The model under review builds one solid part; all positions refer to its coordinate system, in mm. A direction names the side the tool comes from. Coordinates: 2 decimals unless noted, no trailing zeros. Order: outer loops, then holes, each group sorted by start corner. A loop starts at its lowest first (then second) coordinate and runs counter-clockwise, first axis right, second up. Notation, with made-up numbers: M -1,15 L 29,15 A32 cw 29,44 Z; hole C 75.5,9 d9. An arc over 180 degrees is marked long. Answer in a Markdown table with one row per item.
from build123d import *

# Parameters (mm, degrees)
F1_DEPTH  = 9.398
F2_W      = 76.2
F2_H      = 33.274
F3_DEPTH  = 9.398
F4_W      = 76.2
F4_H      = 29.7886691538
F5_DEPTH  = 63.754
F6_SIZE   = 11.43
F7_W      = 76.2
F7_H      = 20.574
F8_DEPTH  = 10.414
F9_R      = 14.224
F10_DEPTH = 58.928


with BuildPart() as f1:
    # F0 (on Top) → F1 (new body)
    with BuildSketch(Plane.XY):
        Polygon((-69.8201261675, 38.4550108689), (-69.8201261675, 21.1263484053), (6.3798738325, 21.1263484053), (6.3798738325, 38.4550108689), (-27.0211261675, 84.4290108689), (-36.4191261675, 84.4290108689), align=None)
    extrude(amount=F1_DEPTH)

    # F2 (on face) → F3 (join)
    with BuildSketch(Plane.XZ.offset(-21.1263484053)):
        with Locations((-31.7201261675, -16.637)):
            Rectangle(F2_W, F2_H)
    extrude(amount=-F3_DEPTH)

    # F4 (on face) → F5 (join)
    with BuildSketch(Plane.XZ.offset(-21.1263484053)):
        with Locations((-31.7201261675, -18.3796654231)):
            Rectangle(F4_W, F4_H)
    extrude(amount=F5_DEPTH)

    # F6
    f6_edges = [f1.edges().sort_by_distance(p)[0] for p in [
        (6.379874, -10.750652, -3.485331),
        (-69.820126, -10.750652, -3.485331),
    ]]
    chamfer(f6_edges, length=F6_SIZE)

    # F7 (on face) → F8 (join)
    with BuildSketch(Plane(origin=(0, 0, -33.274), x_dir=(1, 0, 0), z_dir=(0, 0, -1))):
        with Locations((-31.7201261675, 0.5906515947)):
            Rectangle(F7_W, F7_H)
    extrude(amount=F8_DEPTH)

    # F9 (on face) → F10 (cut)
    with BuildSketch(Plane.XY.offset(-3.4853308462)):
        with Locations((-31.7201261675, -10.7506515947)):
            Circle(F9_R)
    extrude(amount=-F10_DEPTH, mode=Mode.SUBTRACT)


solid = f1.part
(1) Take a section at A-A (y = -20.5). Write out the cut boundary in (x, z), then the cut area to 3 significant figures.
Report:
| item | result |
|---|---|
| outline | M -69.82,-33.27 L -42.08,-33.27 L -42.08,-3.49 L -58.39,-3.49 L -69.82,-14.92 Z; M -21.36,-33.27 L 6.38,-33.27 L 6.38,-14.92 L -5.05,-3.49 L -21.36,-3.49 Z |
| area | 1,520 mm^2 |
(2) Machinability: for faces 5 (the flat face through (-32, 9.696, -38)), 6 (the flat face through (-44, -3, -3.485)), 7 (the flat face through (-6, -10.878, -38)), which of the approach directions +Z, -Z, +X, -X, +Y, -Y give a long, thin tool a straight path to every point of the face, cutting with its end or side? Answer none if there is none.
Report:
| item | result |
|---|---|
| face 5 | -Z, +X, -X, +Y |
| face 6 | +Z, +X, -X, -Y |
| face 7 | -Z, +X, -X, -Y |
(3) Take a section at B-B (z = 6.5). Write out the cut boundary in (x, y).
Report:
| item | result |
|---|---|
| outline | M -69.82,21.13 L 6.38,21.13 L 6.38,38.46 L -27.02,84.43 L -36.42,84.43 L -69.82,38.46 Z |
(4) To check wall thickness, follow line 1 (X direction, y = -10.5, z = -27.5); line 2 (Z direction, x = -54, y = -30.5); line 3 (Y direction, x = -15.5, z = -32). State the ranges of each line that lie inside material, in increasing order. Write a range as [from, to].
Report:
| item | result |
|---|---|
| line 1 | [-69.82, -45.94], [-17.5, 6.38] |
| line 2 | [-33.27, -3.49] |
| line 3 | [-42.63, 30.52] |
(5) The part is to be moulded in two halves that separate along X. For faces 1 (the flat face through (6.38, -2, -23)), 2 (the flat face through (-32, 21.126, 3)), 3 (the cylindrical face through (-33.572, 3.352, -23.305)), 4 (the flat face through (-69.82, -2, -23)), say which applies: +X half, -X half, draft (parallel to the pull), parting line (faces both ways), or undercut.
Report:
| item | result |
|---|---|
| face 1 | +X half |
| face 2 | draft |
| face 3 | undercut |
| face 4 | -X half |
(6) Take a section at D-D (z = -25). Write out the cut boundary in (x, y).
Report:
| item | result |
|---|---|
| outline | M -69.82,-42.63 L 6.38,-42.63 L 6.38,30.52 L -69.82,30.52 Z; hole C -31.72,-10.75 d28.45 |
(7) Take a section at C-C (x = -7). Write out the cut boundary in (y, z), then the cut area to 3 significant figures.
Report:
| item | result |
|---|---|
| outline | M -42.63,-33.27 L -10.88,-33.27 L -10.88,-43.69 L 9.7,-43.69 L 9.7,-33.27 L 30.52,-33.27 L 30.52,0 L 56.87,0 L 56.87,9.4 L 21.13,9.4 L 21.13,-3.49 L -42.63,-3.49 Z |
| area | 2,760 mm^2 |
(8) Insertion check: P1, Ø5, axis at x = -9, z = -36.5, coming from the -Y side; P2, Ø1, axis at x = -36, z = -25, coming from the +Y side; P3, Ø16, axis at x = -40, y = -3.5, coming from the +Z side. Each pin has a flat end and moves straight along its axis. Give the tip position at first contact, or say it passes through.
Report:
| item | result |
|---|---|
| P1 | y = -10.88 |
| P2 | y = 30.52 |
| P3 | z = -3.49 |
